Work out the finished part from the listing and answer in its coordinate system (mm). Face numbers are marked on the shaded views. A direction names the side the tool comes from. Give positions to 0.01 mm unless a question says otherwise; leave off trailing zeros. Write each loop counter-clockwise with the first axis right and the second up, starting at its lowest first coordinate (ties: lowest second). Pieces come first, ordered by that corner, then holes. Notation, with made-up numbers: (43, -18.5) -> (50, -18.5) arc R22 cw to (50, 9.5) -> close; hole circle Ø2 at (-14.75, 31). An arc over 180 degrees is marked (long way). Use a Markdown table: item, result. Add a question column.
Q1. Section B-B, the plane y = 14 is taken. Give the vertices of the cut face in (x, z).
Q2. Section A-A, the plane x = 0 is taken. Give the vertices of the cut face in (y, z), plus the area to 3 significant figures.
Q3. Section C-C, the plane z = 41.5 is taken. Give the vertices of the cut face in (x, y).
Q4. Each of these flat-tipped pins is pushed along its axis until it touches: pin 1 Ø4 at (x, z) = (-15.5, 46) entering from +Y; pin 2 Ø2.5 at (x, y) = (0, 20) entering from -Z; pin 3 Ø6.5 at (x, y) = (0.5, 21) entering from +Z. Where does it stop, or does it pass through?
Q5. Section D-D, the plane x = 10.5 is taken. Give the vertices of the cut face in (y, z).
Q6. For the marked faces 1 and 2, determine the directions among +Z, -Z, +X, -X, +Y, -Y from which every point of the face is accessible in a straight line to the end or side of a thin tool.
Q7. Consider line 1 (Y direction, x = 0, z = -0.5); line 2 (Y direction, x = 2, z = 35); line 3 (Z direction, x = 10.5, y = -14). Determine where each line is inside the solid, lowest interval first.
from build123d import *

# Parameters (mm, degrees)
EXTRUDE_1_DEPTH     = 3
EXTRUDE_2_DEPTH     = 2.5
SKETCH_3_W          = 46.535898384
SKETCH_3_H          = 60
EXTRUDE_3_DEPTH     = 1.5
FILLET_1_R          = 1
SKETCH_4_R          = 1.5
CUT_EXTRUDE_1_DEPTH = 70.387823433


with BuildPart() as part:
    # 草圖1 → 填料-伸長1 (new, symmetric)
    with BuildSketch(Plane.XY):
        with BuildLine():
            ThreePointArc((3.464101615, 10.536922378), (2, 12.001023993), (0, 12.536922378))
            Line((0, 12.536922378), (0, -18.104093774))
            Line((0, -18.104093774), (18.267949192, -18.104093774))
            ThreePointArc((18.267949192, -18.104093774), (19.133974596, -17.604093774), (19.133974596, -16.604093774))
            Line((19.133974596, -16.604093774), (3.464101615, 10.536922378))
        make_face()
        with BuildLine():
            ThreePointArc((0, 12.536922378), (-2, 12.001023993), (-3.464101615, 10.536922378))
            Line((-3.464101615, 10.536922378), (-19.133974596, -16.604093774))
            ThreePointArc((-19.133974596, -16.604093774), (-19.133974596, -17.604093774), (-18.267949192, -18.104093774))
            Line((-18.267949192, -18.104093774), (0, -18.104093774))
            Line((0, -18.104093774), (0, 12.536922378))
        make_face()
    extrude(amount=EXTRUDE_1_DEPTH, both=True)

    # 草圖2 → 填料-伸長2 (add, symmetric)
    with BuildSketch(Plane.XY):
        with BuildLine():
            Line((-3.98839196, 24.947564001), (-3.98839196, 8.841437682))
            Line((-3.98839196, 8.841437682), (3.98839196, 8.841437682))
            Line((3.98839196, 8.841437682), (3.98839196, 24.947564001))
            ThreePointArc((3.98839196, 24.947564001), (3.699590962, 25.65055474), (3, 25.947496625))
            Line((3, 25.947496625), (3, 21.386539183))
            Line((3, 21.386539183), (0, 21.386539183))
            Line((0, 21.386539183), (-3, 21.386539183))
            Line((-3, 21.386539183), (-3, 25.947496625))
            ThreePointArc((-3, 25.947496625), (-3.699590962, 25.65055474), (-3.98839196, 24.947564001))
        make_face()
    extrude(amount=EXTRUDE_2_DEPTH, both=True)

    # 草圖3 → 填料-伸長3 (add)
    with BuildSketch(Plane.XZ.offset(18.104093774)):
        with Locations((0, 27)):
            Rectangle(SKETCH_3_W, SKETCH_3_H)
    extrude(amount=-EXTRUDE_3_DEPTH)

    # 圓角1
    fillet_1_edges = [part.edges().sort_by_distance(p)[0] for p in [
        (19.133974596, -16.604093774, 0),
        (-19.133974596, -16.604093774, 0),
    ]]
    fillet(fillet_1_edges, radius=FILLET_1_R)

    # 草圖4 → 除料-伸長1 (cut, through all)
    with BuildSketch(Plane(origin=(0, 0, -3), x_dir=(-1, 0, 0), z_dir=(0, 0, -1))):
        with Locations((0, 8.536922378)):
            Circle(SKETCH_4_R)
    extrude(amount=-CUT_EXTRUDE_1_DEPTH, mode=Mode.SUBTRACT)


solid = part.part
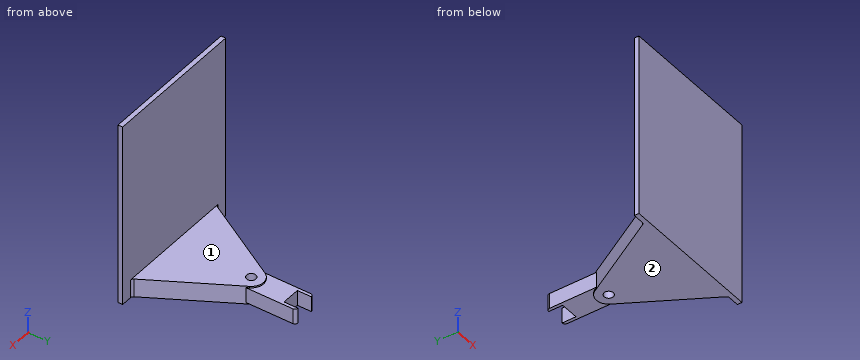
Result set:
| question | item | result |
|---|---|---|
| 1 | outline | (-3.99, -2.5) -> (3.99, -2.5) -> (3.99, 2.5) -> (-3.99, 2.5) -> close |
| 2 | outline | (-18.1, -3) -> (7.04, -3) -> (7.04, 3) -> (-16.6, 3) -> (-16.6, 57) -> (-18.1, 57) -> close; (10.04, -3) -> (12.54, -3) -> (12.54, -2.5) -> (21.39, -2.5) -> (21.39, 2.5) -> (12.54, 2.5) -> (12.54, 3) -> (10.04, 3) -> close |
| 2 | area | 291 mm2 |
| 3 | outline | (-23.27, -18.1) -> (23.27, -18.1) -> (23.27, -16.6) -> (-23.27, -16.6) -> close |
| 4 | pin 1 | stops at y = -16.6 |
| 4 | pin 2 | stops at z = -2.5 |
| 4 | pin 3 | stops at z = 2.5 |
| 5 | outline | (-18.1, -3) -> (-1.65, -3) -> (-1.65, 3) -> (-16.6, 3) -> (-16.6, 57) -> (-18.1, 57) -> close |
| 6 | face 1 | +Z, +X, -X, +Y |
| 6 | face 2 | -Z, +X, -X, +Y, -Y |
| 7 | line 1 | y = -18.1 to 7.04, 10.04 to 21.39 |
| 7 | line 2 | y = -18.1 to -16.6 |
| 7 | line 3 | z = -3 to 3 |
